from build123d import *

# Parameters (mm, degrees)
F0_R      = 31.5
F1_DEPTH  = 22
F3_R      = 14
F4_DEPTH  = 22.001
F5_SIZE   = 9
F6_W      = 15
F6_H      = 8
F7_DEPTH  = 17
F2_R      = 29
F8_DEPTH  = 13
F9_W      = 11.6111175559
F9_H      = 5.5
F10_DEPTH = 5
F11_R     = 2.45
F12_DEPTH = 18.5
F13_W     = 3.3197699547
F13_H     = 4.9
F14_DEPTH = 8
F15_SIZE  = 1


with BuildPart() as f1:
    # F0 (on Top) → F1 (new body)
    with BuildSketch(Plane.XY):
        Circle(F0_R)
    extrude(amount=-F1_DEPTH)

    # F3 (on face) → F4 (cut, through all)
    with BuildSketch(Plane(origin=(0, 0, -22), x_dir=(1, 0, 0), z_dir=(0, 0, -1))):
        Circle(F3_R)
    extrude(amount=-F4_DEPTH, mode=Mode.SUBTRACT)

    # F5
    f5_edges = [f1.edges().sort_by_distance(p)[0] for p in [
        (-31.5, 0, -22),
    ]]
    chamfer(f5_edges, length=F5_SIZE)

    # F6 (on face) → F7 (join)
    with BuildSketch(Plane(origin=(0, 0, -22), x_dir=(1, 0, 0), z_dir=(0, 0, -1))):
        with Locations((29, 0)):
            Rectangle(F6_W, F6_H)
        Polygon((21.7141016151, 29.6099272381), (14.7858983849, 33.6099272381), (7.2858983849, 20.6195461814), (14.2141016151, 16.6195461814), align=None)
        Polygon((-14.7858983849, 33.6099272381), (-21.7141016151, 29.6099272381), (-14.2141016151, 16.6195461814), (-7.2858983849, 20.6195461814), align=None)
        with Locations((-29, 0)):
            Rectangle(F6_W, F6_H)
        Polygon((-21.7141016151, -29.6099272381), (-14.7858983849, -33.6099272381), (-7.2858983849, -20.6195461814), (-14.2141016151, -16.6195461814), align=None)
        Polygon((14.7858983849, -33.6099272381), (21.7141016151, -29.6099272381), (14.2141016151, -16.6195461814), (7.2858983849, -20.6195461814), align=None)
    extrude(amount=-F7_DEPTH)

    # F2 (on face) → F8 (cut)
    with BuildSketch(Plane.XY):
        Circle(F2_R)
    extrude(amount=-F8_DEPTH, mode=Mode.SUBTRACT)

    # F9 (on face) → F10 (cut)
    with BuildSketch(Plane.XY):
        with Locations((30.3034381941, 0)):
            Rectangle(F9_W, F9_H)
        Polygon((20.4360683464, 29.896308683), (15.6729286256, 32.646308683), (9.8673698477, 22.5907859132), (14.6305095685, 19.8407859132), align=None)
        Polygon((-15.6729286256, 32.646308683), (-20.4360683464, 29.896308683), (-14.6305095685, 19.8407859132), (-9.8673698477, 22.5907859132), align=None)
        with Locations((-30.3034381941, 0)):
            Rectangle(F9_W, F9_H)
        Polygon((-20.4360683464, -29.896308683), (-15.6729286256, -32.646308683), (-9.8673698477, -22.5907859132), (-14.6305095685, -19.8407859132), align=None)
        Polygon((15.6729286256, -32.646308683), (20.4360683464, -29.896308683), (14.6305095685, -19.8407859132), (9.8673698477, -22.5907859132), align=None)
    extrude(amount=-F10_DEPTH, mode=Mode.SUBTRACT)

    # F11 (on face) → F12 (join)
    with BuildSketch(Plane.XY.offset(-13)):
        with Locations((-26.4, 0)):
            Circle(F11_R)
        with Locations((-13.2, -22.8630706599)):
            Circle(F11_R)
        with Locations((13.2, -22.8630706599)):
            Circle(F11_R)
        with Locations((26.4, 0)):
            Circle(F11_R)
        with Locations((13.2, 22.8630706599)):
            Circle(F11_R)
        with Locations((-13.2, 22.8630706599)):
            Circle(F11_R)
    extrude(amount=F12_DEPTH)

    # F13 (on face) → F14 (join)
    with BuildSketch(Plane.XY.offset(-13)):
        with Locations((-28.0598849773, 0)):
            Rectangle(F13_W, F13_H)
        Polygon((-16.9816472166, -24.5130757754), (-12.7381227381, -26.9630757754), (-11.0782377607, -24.0880706599), (-15.3217622393, -21.6380706599), align=None)
        Polygon((12.7381227381, -26.9630757754), (16.9816472166, -24.5130757754), (15.3217622393, -21.6380706599), (11.0782377607, -24.0880706599), align=None)
        with Locations((28.0598849773, 0)):
            Rectangle(F13_W, F13_H)
        Polygon((16.9816472166, 24.5130757754), (12.7381227381, 26.9630757754), (11.0782377607, 24.0880706599), (15.3217622393, 21.6380706599), align=None)
        Polygon((-12.7381227381, 26.9630757754), (-16.9816472166, 24.5130757754), (-15.3217622393, 21.6380706599), (-11.0782377607, 24.0880706599), align=None)
    extrude(amount=F14_DEPTH)

    # F15
    f15_edges = [f1.edges().sort_by_distance(p)[0] for p in [
        (-14, 0, -22),
        (-14, 0, -13),
        (-18.124499, -23.392553, -22),
        (-11.196296, -27.392553, -22),
        (11.196296, -27.392553, -22),
        (18.124499, -23.392553, -22),
        (29.320795, -4, -22),
        (29.320795, 4, -22),
        (18.124499, 23.392553, -22),
        (11.196296, 27.392553, -22),
        (-11.196296, 27.392553, -22),
        (-18.124499, 23.392553, -22),
        (-29.320795, 4, -22),
        (-29.320795, -4, -22),
    ]]
    chamfer(f15_edges, length=F15_SIZE)


solid = f1.part
Geometry: final body of the model. Coordinates: model frame, mm. A direction names the side the tool comes from. Give positions to 0.01 mm unless a question says otherwise; leave off trailing zeros. Write each loop counter-clockwise with the first axis right and the second up, starting at its lowest first coordinate (ties: lowest second). Pieces come first, ordered by that corner, then holes. Notation, with made-up numbers: M 35.5,-15.75 L 40.5,-15.75 A18 cw 40.5,4.25 Z; hole C -38.75,78 d8. An arc over 180 degrees is marked long. Answer in a Markdown table with one row per item. Add a question column.
(1) Section D-D on z = 2.5. Return loops of the section in (x, y).
(2) Section C-C on x = 20. State how many separate pieces and enclosed holes the cut face has, and give its area (3 significant figures).
(3) Reachability of faces 4 (the flat face through (26, 14, 0)), 5 (the cylindrical face through (-11.88, -20.8, -1.82)), 6 (the flat face through (-0.2, -29.5, 0)), 7 (the flat face through (33, -4, -15)), 8 (the flat face through (-19.814, 26.319, -14.89)) from +Z, -Z, +X, -X, +Y, -Y: full face, straight path, thin tool, end or side. Return the list, or none.
(4) First-contact query: pin 1 (4.5 mm diameter, centred on x = -26, y = 9.5, fed in from +Z); pin 2 (3 mm diameter, centred on y = 10.5, z = 2.5, fed in from +X); pin 3 (3 mm diameter, centred on x = 16, y = 30.5, fed in from +Z); pin 4 (3 mm diameter, centred on x = -30.5, z = -2.5, fed in from +Y). Flat tips, straight axial feed; report the tip coordinate or a pass-through.
(5) Mould query, pull axis X, two halves, no side actions, for faces 1 (the conical face through (-23.253, 13.598, -17.563)), 2 (the flat face through (13, -23, 5.5)), 3 (the flat face through (-28, -2.45, -9)). Classes: +X half, -X half, draft (parallel to the pull), parting line (faces both ways), or undercut.
(6) Section A-A on y = 0. Return loops of the section in (x, z).
(7) Ray query, line 1 (X direction, y = 0, z = -16.75); line 2 (Y direction, x = -33, z = -14); line 3 (Y direction, x = 0, z = -19.5). Return the intervals inside material, ascending.
(8) Section B-B on z = -15. Return loops of the section in (x, y), and give its area (3 significant figures).
Result set:
| question | item | result |
|---|---|---|
| 1 | outline | C -26.4,0 d4.9; C -13.2,-22.86 d4.9; C -13.2,22.86 d4.9; C 13.2,-22.86 d4.9; C 13.2,22.86 d4.9; C 26.4,0 d4.9 |
| 2 | separate pieces | 3 |
| 2 | enclosed holes | 0 |
| 2 | area | 541 mm^2 |
| 3 | face 4 | +Z, +X, +Y |
| 3 | face 5 | +Z |
| 3 | face 6 | +Z, +X, -X, -Y |
| 3 | face 7 | -Z, +X, -Y |
| 3 | face 8 | -Z, -X |
| 4 | pin 1 | stops at z = 0 |
| 4 | pin 2 | passes through |
| 4 | pin 3 | stops at z = -5 |
| 4 | pin 4 | stops at y = 12.3 |
| 5 | face 1 | -X half |
| 5 | face 2 | draft |
| 5 | face 3 | undercut |
| 6 | outline | M -36.5,-22 L -15,-22 L -14,-21 L -14,-14 L -15,-13 L -23.95,-13 L -23.95,5.5 L -28.85,5.5 L -28.85,-5 L -36.5,-5 Z; M 14,-21 L 15,-22 L 36.5,-22 L 36.5,-5 L 28.85,-5 L 28.85,5.5 L 23.95,5.5 L 23.95,-13 L 15,-13 L 14,-14 Z |
| 7 | line 1 | x = -36.5 to -14, 14 to 36.5 |
| 7 | line 2 | y = -4 to 4 |
| 7 | line 3 | y = -25 to -14, 14 to 25 |
| 8 | outline | M -36.5,-4 L -29.23,-4 A29.5 ccw -18.08,-23.31 L -21.71,-29.61 L -14.79,-33.61 L -11.15,-27.31 A29.5 ccw 11.15,-27.31 L 14.79,-33.61 L 21.71,-29.61 L 18.08,-23.31 A29.5 ccw 29.23,-4 L 36.5,-4 L 36.5,4 L 29.23,4 A29.5 ccw 18.08,23.31 L 21.71,29.61 L 14.79,33.61 L 11.15,27.31 A29.5 ccw -11.15,27.31 L -14.79,33.61 L -21.71,29.61 L -18.08,23.31 A29.5 ccw -29.23,4 L -36.5,4 Z; hole C 0,0 d28 |
| 8 | area | 2,460 mm^2 |
